Part print with two shaded views. Sizes in mm from the minimum x, y, z corner. Coordinates: 2 decimals unless noted, no trailing zeros. Order: outer loops, then holes, each group sorted by start corner. A loop starts at its lowest first (then second) coordinate and runs counter-clockwise, first axis right, second up. Notation, with made-up numbers: (56, 66.25) - (102, 66.25) arc R19 cw to (102, 99.25) - close; hole circle Ø1 at (60, 62.5). An arc over 180 degrees is marked (long way). Return JSON: item names as keys, results as strings.
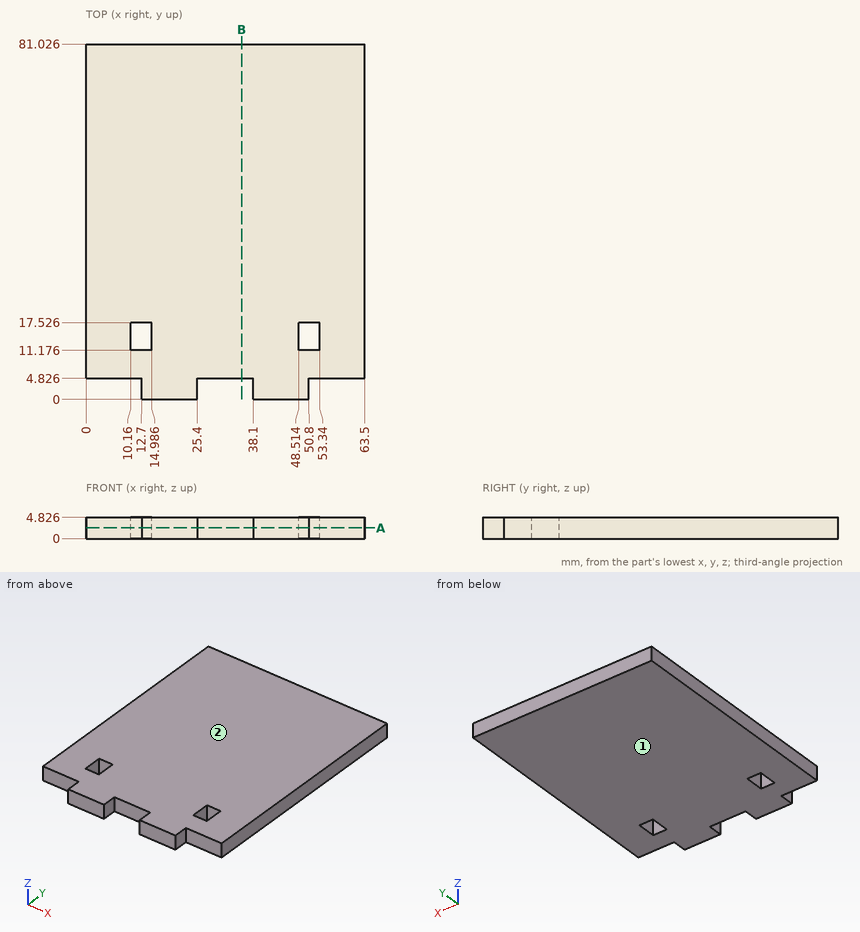
Item 1: Band-saw the part on B-B, the plane x = 35.5. List the corners of the cut face in (y, z).
Findings below:
{"outline": "(4.83, 0) - (81.03, 0) - (81.03, 4.83) - (4.83, 4.83) - close"}
Item 2: Band-saw the part on A-A, the plane z = 2.45. List the corners of the cut face in (x, y).
Findings below:
{"outline": "(0, 4.83) - (12.7, 4.83) - (12.7, 0) - (25.4, 0) - (25.4, 4.83) - (38.1, 4.83) - (38.1, 0) - (50.8, 0) - (50.8, 4.83) - (63.5, 4.83) - (63.5, 81.03) - (0, 81.03) - close; hole (10.16, 11.18) - (14.99, 11.18) - (14.99, 17.53) - (10.16, 17.53) - close; hole (48.51, 11.18) - (53.34, 11.18) - (53.34, 17.53) - (48.51, 17.53) - close"}
Item 3: Mould opens along Z. For the marked faces 1 and 2 say: released by +Z, released by -Z, zero draft, split by the parting line, or undercut.
Findings below:
{"face 1": "released by -Z", "face 2": "released by +Z"}
Item 4: Drop flat-ended pins along their axis: P1, Ø1.4, axis at y = 2.5, z = 3, coming from the +X side; P2, Ø1.4, axis at y = 1.5, z = 3, coming from the -X side; P3, Ø2, axis at x = 10.5, z = 1.5, coming from the -Y side. Give the stop position or say it passes through.
Findings below:
{"P1": "stops at x = 50.8", "P2": "stops at x = 12.7", "P3": "stops at y = 4.83"}
Item 5: Wall check: L1, parallel to X at y = 4, z = 1.1; L2, parallel to Y at x = 11.5, z = 3.7; L3, parallel to Y at x = 26.5, z = 1.1. Give the ranges that are in metal, low to high. Write a range as [from, to].
Findings below:
{"L1": "x = [12.7, 25.4], [38.1, 50.8]", "L2": "y = [4.83, 11.18], [17.53, 81.03]", "L3": "y = [4.83, 81.03]"}
